Work out the finished part from the listing and answer in its coordinate system (mm). A direction names the side the tool comes from. Give positions to 0.01 mm unless a question says otherwise; leave off trailing zeros. Loops run counter-clockwise (first coordinate to the right, second up) from the corner with the lowest first, then second, coordinate; pieces in that order, holes last. Notation, with made-up numbers: M -32,47.5 L -2,47.5 A10 cw -2,52.5 Z; hole C 63,52 d6. An arc over 180 degrees is marked long. Answer as a JSON object with one key per item and string values. Group by question number.
```python
from build123d import *

# Parameters (mm, degrees)
REVOLVE1_START                       = -42
REVOLVE1_DEPTH                       = 42
REVOLVE1_2_DEPTH                     = 10
REVOLVE1_START_2                     = -32
REVOLVE1_3_DEPTH                     = 12
SKETCH2_R                            = 3
BOSS_EXTRUDE1_DEPTH                  = 6
BOSS_EXTRUDE1_DIRECTION_2_REACH      = 66.094
BOSS_EXTRUDE1_DIRECTION_2_END_RADIUS = 30


# Read off the part's stored shape, not the designer's step: Revolve1
with BuildPart() as part:
    # Revolve1 outline → Revolve1 (new body)
    with BuildSketch(Plane.XY.offset(REVOLVE1_START)):
        with BuildLine():
            ThreePointArc((-25, 0), (0, 25), (25, 0))
            Line((25, 0), (30, 0))
            ThreePointArc((30, 0), (0, 30), (-30, 0))
            Line((-30, 0), (-25, 0))
        make_face()
    revolve1 = extrude(amount=REVOLVE1_DEPTH)



with BuildPart() as body_2:
    # Revolve1 2 outline → Revolve1 2 (new body)
    with BuildSketch(Plane.XY.offset(REVOLVE1_START)):
        with BuildLine():
            ThreePointArc((-30, 0), (0, 30), (30, 0))
            Line((30, 0), (38, 0))
            ThreePointArc((38, 0), (0, 38), (-38, 0))
            Line((-38, 0), (-30, 0))
        make_face()
    revolve1_2 = extrude(amount=REVOLVE1_2_DEPTH)


with BuildPart() as part_1:
    add(part.part)

    add(body_2.part)  # Revolve1 3 merges body 2
    # Revolve1 3 outline → Revolve1 3 (add)
    with BuildSketch(Plane.XY.offset(REVOLVE1_START_2)):
        with BuildLine():
            ThreePointArc((-30, 0), (0, 30), (30, 0))
            Line((30, 0), (32, 0))
            ThreePointArc((32, 0), (0, 32), (-32, 0))
            Line((-32, 0), (-30, 0))
        make_face()
    revolve1_3 = extrude(amount=REVOLVE1_3_DEPTH)

    # Mirror1: Revolve1, Revolve1 2, Revolve1 3 across plane
    add(revolve1.mirror(Plane(origin=(30, 0, 0), x_dir=(1, 0, 0), z_dir=(0, 0, -1))))
    add(revolve1_2.mirror(Plane(origin=(30, 0, 0), x_dir=(1, 0, 0), z_dir=(0, 0, -1))))
    add(revolve1_3.mirror(Plane(origin=(30, 0, 0), x_dir=(1, 0, 0), z_dir=(0, 0, -1))))

    # Sketch2 → Boss-Extrude1 (add)
    with BuildSketch(Plane(origin=(0, 30, 0), x_dir=(1, 0, 0), z_dir=(0, 1, 0))):
        with Locations(Location((0, 0, 0), (0, 0, 90))):
            Circle(SKETCH2_R)
    extrude(amount=BOSS_EXTRUDE1_DEPTH)

    # Boss-Extrude1 direction 2: up to this cylinder (the profile starts outside it)
    boss_extrude1_direction_2_end = Plane(origin=(0, 0, 0), z_dir=(0, 0, 1)) * Cylinder(BOSS_EXTRUDE1_DIRECTION_2_END_RADIUS, 193.188, mode=Mode.PRIVATE)
    # Sketch2 → Boss-Extrude1 direction 2 (add, up to the surface)
    with BuildSketch(Plane(origin=(0, 30, 0), x_dir=(1, 0, 0), z_dir=(0, 1, 0)), mode=Mode.PRIVATE) as boss_extrude1_direction_2_sk1:
        with Locations(Location((0, 0, 0), (0, 0, 90))):
            Circle(SKETCH2_R)
    boss_extrude1_direction_2_tool1 = extrude(boss_extrude1_direction_2_sk1.sketch, amount=-BOSS_EXTRUDE1_DIRECTION_2_REACH, mode=Mode.PRIVATE) - boss_extrude1_direction_2_end
    add(boss_extrude1_direction_2_tool1.solids().sort_by_distance((0, 30, 0))[0])
    add(boss_extrude1_direction_2_tool1.solids().sort_by_distance((0, 30, 0))[1])


solid = part_1.part
```
Item 1: A cutting plane is placed at C-C (y = 4). Determine the outline of the cut face in (x, z), and give its area (3 significant figures).
Item 2: Given pin 1 Ø2 at (x, z) = (29.5, 19.5) entering from +Y; pin 2 Ø8 at (x, z) = (0, -12) entering from +Y; pin 3 Ø1 at (y, z) = (18, 5.5) entering from -X, each flat-ended and moving along its own axis, determine where each tip first touches the part or whether it passes through.
Item 3: A cutting plane is placed at B-B (z = 0). Determine the outline of the cut face in (x, y), and give its area (3 significant figures).
Item 4: Find the intervals of material crossed by probe 1 along Z at (x, y) = (7, 32); probe 2 along Z at (x, y) = (-5, 30.5); probe 3 along Z at (x, y) = (-2.5, 30), in increasing order. Write a range as [from, to].
Item 5: A tool of negligible diameter and unlimited length cuts with its end or side. For faces 5 (the flat face through (0, 36, 0)), 6 (the flat face through (-0.1, 30.3, 20)), 7 (the cylindrical face through (0.84, 37.99, -37.07)), from which of +Z, -Z, +X, -X, +Y, -Y can it reach the whole face along a straight path? Write none if from no direction.
Item 6: A cutting plane is placed at D-D (x = -9). Determine the outline of the cut face in (y, z), and give its area (3 significant figures).
Item 7: A cutting plane is placed at A-A (x = 33). Determine the outline of the cut face in (y, z), and give its area (3 significant figures).
Item 8: For a pull along Z with two mould halves and no side action, classify faces 1 (the flat face through (-0.1, 30.3, -20)), 2 (the flat face through (-1, 28, 42)), 3 (the flat face through (-1, 28, -42)), 4 (the cylindrical face through (0.84, 37.99, 37.07)) as pulls with the +Z half, pulls with the -Z half, needs draft (parallel to the pull), parting line crosses it, or undercut.
The answers:
{
 "1": {"outline": "M -37.79,-42 L -24.68,-42 L -24.68,42 L -37.79,42 L -37.79,32 L -31.75,32 L -31.75,20 L -29.73,20 L -29.73,-20 L -31.75,-20 L -31.75,-32 L -37.79,-32 Z; M 24.68,-42 L 37.79,-42 L 37.79,-32 L 31.75,-32 L 31.75,-20 L 29.73,-20 L 29.73,20 L 31.75,20 L 31.75,32 L 37.79,32 L 37.79,42 L 24.68,42 Z", "area": "1,270 mm^2"},
 "2": {"pin 1": "stops at y = 14.29", "pin 2": "stops at y = 30", "pin 3": "stops at x = -24.37"},
 "3": {"outline": "M -30,0 L -25,0 A25 cw 25,0 L 30,0 A30 ccw 3,29.85 L 3,36 L -3,36 L -3,29.85 A30 ccw Z", "area": "468 mm^2"},
 "4": {"probe 1": "z = [-42, -32], [32, 42]", "probe 2": "z = [-42, -20], [20, 42]", "probe 3": "z = [-42, -20], [-1.66, 1.66], [20, 42]"},
 "5": {"face 5": "+X, -X, +Y", "face 6": "+Y", "face 7": "+Z, -Z, +Y"},
 "6": {"outline": "M 23.32,-42 L 36.92,-42 L 36.92,-32 L 30.71,-32 L 30.71,-20 L 28.62,-20 L 28.62,20 L 30.71,20 L 30.71,32 L 36.92,32 L 36.92,42 L 23.32,42 Z", "area": "661 mm^2"},
 "7": {"outline": "M 0,-42 L 18.84,-42 L 18.84,-32 L 0,-32 Z; M 0,32 L 18.84,32 L 18.84,42 L 0,42 Z", "area": "377 mm^2"},
 "8": {"face 1": "undercut", "face 2": "pulls with the +Z half", "face 3": "pulls with the -Z half", "face 4": "needs draft"}
}
